Geometry: final body of the model. Coordinates: model frame, mm. Give positions to 0.01 mm unless a question says otherwise; leave off trailing zeros. Write each loop counter-clockwise with the first axis right and the second up, starting at its lowest first coordinate (ties: lowest second). Pieces come first, ordered by that corner, then holes.
Q1. Section D-D (x = -4.5). Return the cut outline in (y, z).
Q2. Section B-B (y = 0). Return the cut outline in (x, z), plus the area to 3 significant figures.
Q3. Mould query, pull axis Y, two halves, no side actions, for faces 1 (the flat face through (8, -25, 25)), 2 (the cylindrical face through (5.015, -0.66, 24.2)), 3 (the flat face through (35.3, -0.4, 0)). Classes: +Y half, -Y half, draft (parallel to the pull), parting line (faces both ways), or undercut.
Q4. Section A-A (x = 20). Return the cut outline in (y, z).
Q5. Pin query (flat end, axial travel): pin 1 Ø3 at (y, z) = (8, 13.5) entering from -X; pin 2 Ø18 at (x, y) = (20, 0) entering from +Z; pin 3 Ø5 at (x, y) = (16, 18.5) entering from -Z; pin 4 Ø4 at (y, z) = (5.5, 12) entering from -X. Return the tip coordinate at first contact, or that it passes through.
Q6. Line query: line 1 (Y direction, x = 20, z = 21); line 2 (X direction, y = 0, z = 27); line 3 (X direction, y = 0, z = 15.5). Output: solid intervals per line, ascending.
Q7. Section C-C (z = 29). Return the cut outline in (x, y), plus the area to 3 significant figures.
from build123d import *

# Parameters (mm, degrees)
F1_DEPTH = 25
F2_R     = 15
F3_DEPTH = 49.087306


with BuildPart() as f1:
    # F0 (on Front) → F1 (new body, symmetric)
    with BuildSketch(Plane.XZ):
        Polygon((-44.064272, 49.086306), (0, 0), (42.768266, 0), (42.768266, 49.086306), align=None)
    extrude(amount=F1_DEPTH, both=True)

    # F2 (on face) → F3 (cut, through all)
    with BuildSketch(Plane(origin=(0, 0, 0), x_dir=(1, 0, 0), z_dir=(0, 0, -1))):
        with Locations((20, 0)):
            Circle(F2_R)
    extrude(amount=-F3_DEPTH, mode=Mode.SUBTRACT)


solid = f1.part
Computed:
1. outline: (-25, 5.01) - (25, 5.01) - (25, 49.09) - (-25, 49.09) - close
2. outline: (-44.06, 49.09) - (0, 0) - (5, 0) - (5, 49.09) - close; (35, 0) - (42.77, 0) - (42.77, 49.09) - (35, 49.09) - close
2. area: 1,710 mm2
3. face 1: -Y half
3. face 2: undercut
3. face 3: draft
4. outline: (-25, 0) - (-15, 0) - (-15, 49.09) - (-25, 49.09) - close; (15, 0) - (25, 0) - (25, 49.09) - (15, 49.09) - close
5. pin 1: stops at x = -13.47
5. pin 2: passes through
5. pin 3: stops at z = 0
5. pin 4: stops at x = -12.57
6. line 1: y = -25 to -15, 15 to 25
6. line 2: x = -24.24 to 5, 35 to 42.77
6. line 3: x = -13.91 to 5, 35 to 42.77
7. outline: (-26.03, -25) - (42.77, -25) - (42.77, 25) - (-26.03, 25) - close; hole circle Ø30 at (20, 0)
7. area: 2,730 mm2
